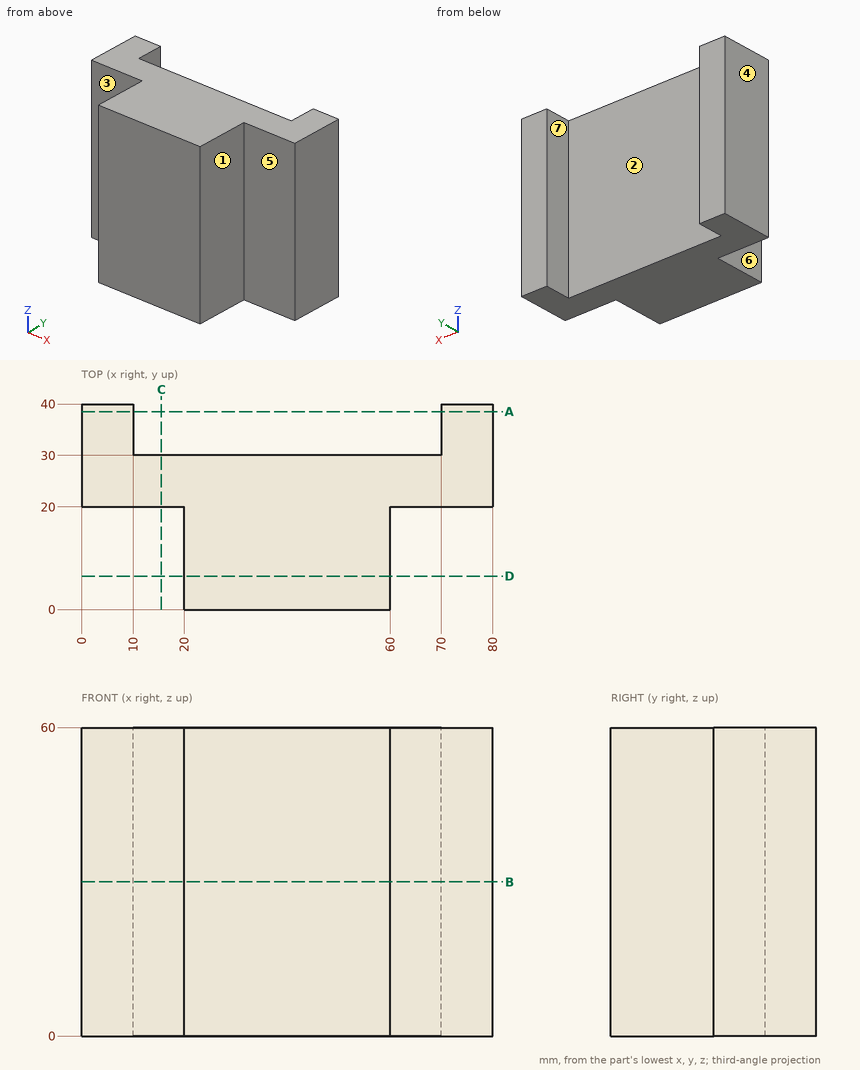
Design review of the part shown in the three views and the two pictorial views. Dimensions are in mm from the part's minimum x, y and z. A direction names the side the tool comes from. Give positions to 0.01 mm unless a question says otherwise; leave off trailing zeros. Write each loop counter-clockwise with the first axis right and the second up, starting at its lowest first coordinate (ties: lowest second). Pieces come first, ordered by that corner, then holes. Notation, with made-up numbers: M 61.5,38 L 110.5,38 A25 ccw 110.5,70 Z; hole C 19.5,12 d5. An arc over 180 degrees is marked long. Return JSON: item names as keys, results as strings. Group by question number.
Item 1: Take a section at B-B (z = 30). Give the boundary of the cut face in (x, y).
Item 2: Take a section at C-C (x = 15.5). Give the boundary of the cut face in (y, z), plus the area to 3 significant figures.
Item 3: Clearance check with flat-ended pins moving along their axes: pin 1 Ø6 at (y, z) = (9, 29.5) entering from +X; pin 2 Ø6 at (x, z) = (10, 21.5) entering from -Y; pin 3 Ø5 at (y, z) = (10.5, 12) entering from -X. State where each tip first meets the part, or that it passes through.
Item 4: Wall thickness on line 1 along X through (y, z) = (34, 51.5); line 2 along Y through (x, z) = (22.5, 14); line 3 along Y through (x, z) = (13.5, 15): over which ranges is each line inside the solid? List them lowest first.
Item 5: The part is to be moulded in two halves that separate along X. For the marked faces 1, 2, 3 and 4, say which applies: pulls with the +X half, pulls with the -X half, needs draft (parallel to the pull), parting line crosses it, or undercut.
Item 6: Take a section at A-A (y = 38.5). Give the boundary of the cut face in (x, z), plus the area to 3 significant figures.
Item 7: Tool access review of the marked faces 5, 6 and 7: name each direction out of +Z, -Z, +X, -X, +Y, -Y from which nothing blocks a thin tool from reaching the whole face with its end or side.
Item 8: Take a section at D-D (y = 6.5). Give the boundary of the cut face in (x, z).
Return value:
{
 "1": {"outline": "M 0,20 L 20,20 L 20,0 L 60,0 L 60,20 L 80,20 L 80,40 L 70,40 L 70,30 L 10,30 L 10,40 L 0,40 Z"},
 "2": {"outline": "M 20,0 L 30,0 L 30,60 L 20,60 Z", "area": "600 mm2"},
 "3": {"pin 1": "stops at x = 60", "pin 2": "stops at y = 20", "pin 3": "stops at x = 20"},
 "4": {"line 1": "x = 0 to 10, 70 to 80", "line 2": "y = 0 to 30", "line 3": "y = 20 to 30"},
 "5": {"face 1": "pulls with the +X half", "face 2": "undercut", "face 3": "needs draft", "face 4": "pulls with the -X half"},
 "6": {"outline": "M 0,0 L 10,0 L 10,60 L 0,60 Z; M 70,0 L 80,0 L 80,60 L 70,60 Z", "area": "1,200 mm2"},
 "7": {"face 5": "+Z, -Z, +X, -Y", "face 6": "+Z, -Z, -X, -Y", "face 7": "+Z, -Z, +Y"},
 "8": {"outline": "M 20,0 L 60,0 L 60,60 L 20,60 Z"}
}
